Part model, mm, in its own coordinate system. Face numbers are marked on the shaded views. A direction names the side the tool comes from. Give positions to 0.01 mm unless a question says otherwise; leave off trailing zeros. Order: outer loops, then holes, each group sorted by start corner. A loop starts at its lowest first (then second) coordinate and runs counter-clockwise, first axis right, second up. Notation, with made-up numbers: (82, 40) - (93, 40) arc R30 ccw to (93, 69) - close; hole circle Ø3 at (49.5, 60.25). An arc over 180 degrees is marked (long way). One line per item, written item: value.
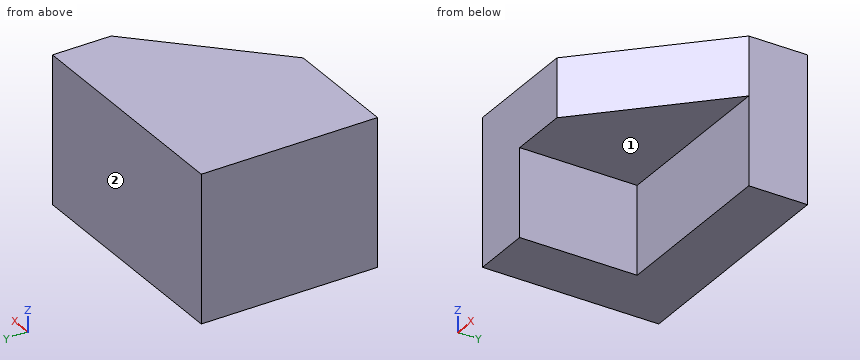
```python
from build123d import *

# Parameters (mm, degrees)
F0_W     = 203.2
F0_H     = 127
F1_DEPTH = 50.8
F2_W     = 50.8
F2_H     = 76.2
F2_H_2   = 50.8
F3_DEPTH = 101.6
F5_DEPTH = 50.8


with BuildPart() as f1:
    # F0 (on Front) → F1 (new body)
    with BuildSketch(Plane.XZ):
        with Locations((-31.441638, 8.165119)):
            Rectangle(F0_W, F0_H)
    extrude(amount=F1_DEPTH)

    # F2 (on face) → F3 (join)
    with BuildSketch(Plane.XZ.offset(50.8)):
        with Locations((-107.641638, -17.234881)):
            Rectangle(F2_W, F2_H)
        with Locations((-107.641638, 46.265119)):
            Rectangle(F2_W, F2_H_2)
        with Locations((-56.841638, 46.265119)):
            Rectangle(F2_W, F2_H_2)
    extrude(amount=F3_DEPTH)

    # F4 (on face) → F5 (join)
    with BuildSketch(Plane.XY.offset(71.665119)):
        Polygon((-31.441638, -50.8), (-31.441638, -152.4), (70.158362, -50.8), align=None)
    extrude(amount=-F5_DEPTH)


solid = f1.part
```
1) Wall check: line 1 along X through (y, z) = (-142.5, 9); line 2 along Y through (x, z) = (-13, -24); line 3 along Z through (x, y) = (-9.5, -114). Give the ranges that are in metal, low to high. Write a range as [from, to].
Answer:
line 1: x = [-133.04, -82.24]
line 2: y = [-50.8, 0]
line 3: z = [20.87, 71.67]
2) Slice it at B-B on x = -6.5. Write the cut outline in (y, z).
Answer:
outline: (-127.46, 20.87) - (-50.8, 20.87) - (-50.8, -55.33) - (0, -55.33) - (0, 71.67) - (-127.46, 71.67) - close
3) Drop flat-ended pins along their axis: P1, Ø1.5, axis at x = -49.5, y = -134, coming from the -Z side; P2, Ø23, axis at y = -122.5, z = -2, coming from the +X side; P3, Ø4, axis at x = 19.5, z = -22.5, coming from the -Y side. Give the stop position or say it passes through.
Answer:
P1: stops at z = 20.87
P2: stops at x = -82.24
P3: stops at y = -50.8
4) Which spindle directions (+Z, -Z, +X, -X, +Y, -Y) get a long thin tool onto all of the face, cutting with end or side? Do the marked faces 1 and 2. Say none if no direction does.
Answer:
face 1: -Z, +X, -Y
face 2: +Z, -Z, +X, -X, +Y
5) Slice it at C-C on z = 31. Write the cut outline in (x, y).
Answer:
outline: (-133.04, -152.4) - (-31.44, -152.4) - (70.16, -50.8) - (70.16, 0) - (-133.04, 0) - close
6) Slice it at A-A on z = -1.5. Write the cut outline in (x, y), then the cut area to 3 significant figures.
Answer:
outline: (-133.04, -152.4) - (-82.24, -152.4) - (-82.24, -50.8) - (70.16, -50.8) - (70.16, 0) - (-133.04, 0) - close
area: 15,500 mm2
